Design review of the part shown in the three views and the two pictorial views. Dimensions are in mm from the part's minimum x, y and z. Round coordinates to 2 decimals unless told otherwise and drop trailing zeros. Loops run counter-clockwise (first coordinate to the right, second up) from the corner with the lowest first, then second, coordinate; pieces in that order, holes last. Notation, with made-up numbers: (-40, 44.25) -> (0, 44.25) arc R38 cw to (0, 83.25) -> close; hole circle Ø11 at (9.5, 1). An arc over 180 degrees is marked (long way). Write each question's results on one line, items separated by ' | '. Start each with the question number.
Item 1: We need section B-B (x = 12.5). Give the boundary of the cut face in (y, z).
Item 2: For L1, parallel to Y at x = 62.5, z = 1.15; L2, parallel to X at y = 13.5, z = 1.45; L3, parallel to Y at x = 59.5, z = 0.8, list the stretches that pass through material, from the lowest coordinate up. Write a range as from..to.
Item 3: We need section A-A (z = 3.7). Give the boundary of the cut face in (x, y).
Item 4: Clearance check with flat-ended pins moving along their axes: pin 1 Ø6.5 at (x, y) = (12.5, 12.5) entering from -Z; pin 2 Ø1 at (x, z) = (66, 4) entering from -Y. State where each tip first meets the part, or that it passes through.
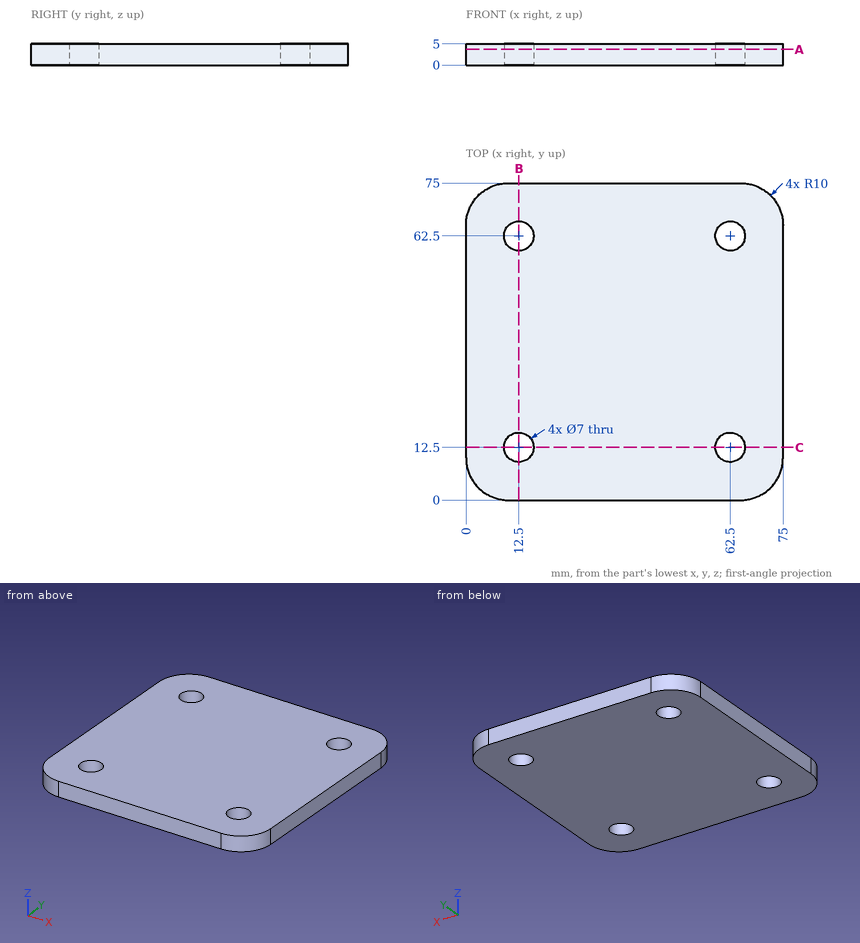
Here are the results:
1) outline: (0, 0) -> (9, 0) -> (9, 5) -> (0, 5) -> close; (16, 0) -> (59, 0) -> (59, 5) -> (16, 5) -> close; (66, 0) -> (75, 0) -> (75, 5) -> (66, 5) -> close
2) L1: y = 0..9, 16..59, 66..75 | L2: x = 0..9.15, 15.85..59.15, 65.85..75 | L3: y = 0..10.7, 14.3..60.7, 64.3..75
3) outline: (0, 10) arc R10 ccw to (10, 0) -> (65, 0) arc R10 ccw to (75, 10) -> (75, 65) arc R10 ccw to (65, 75) -> (10, 75) arc R10 ccw to (0, 65) -> close; hole circle Ø7 at (12.5, 12.5); hole circle Ø7 at (12.5, 62.5); hole circle Ø7 at (62.5, 12.5); hole circle Ø7 at (62.5, 62.5)
4) pin 1: passes through | pin 2: stops at y = 0.01
